Check sheet for the drawn part. Datum: minimum x, y, z corner. Units: mm. Coordinates: 2 decimals unless noted, no trailing zeros. Order: outer loops, then holes, each group sorted by start corner. A loop starts at its lowest first (then second) coordinate and runs counter-clockwise, first axis right, second up. Notation, with made-up numbers: (-32.75, 46) - (24.25, 46) arc R22 cw to (24.25, 57) - close; hole circle Ø3 at (-3, 79.5). An arc over 180 degrees is marked (long way). One line per item, written item: value. Start each with the question number.
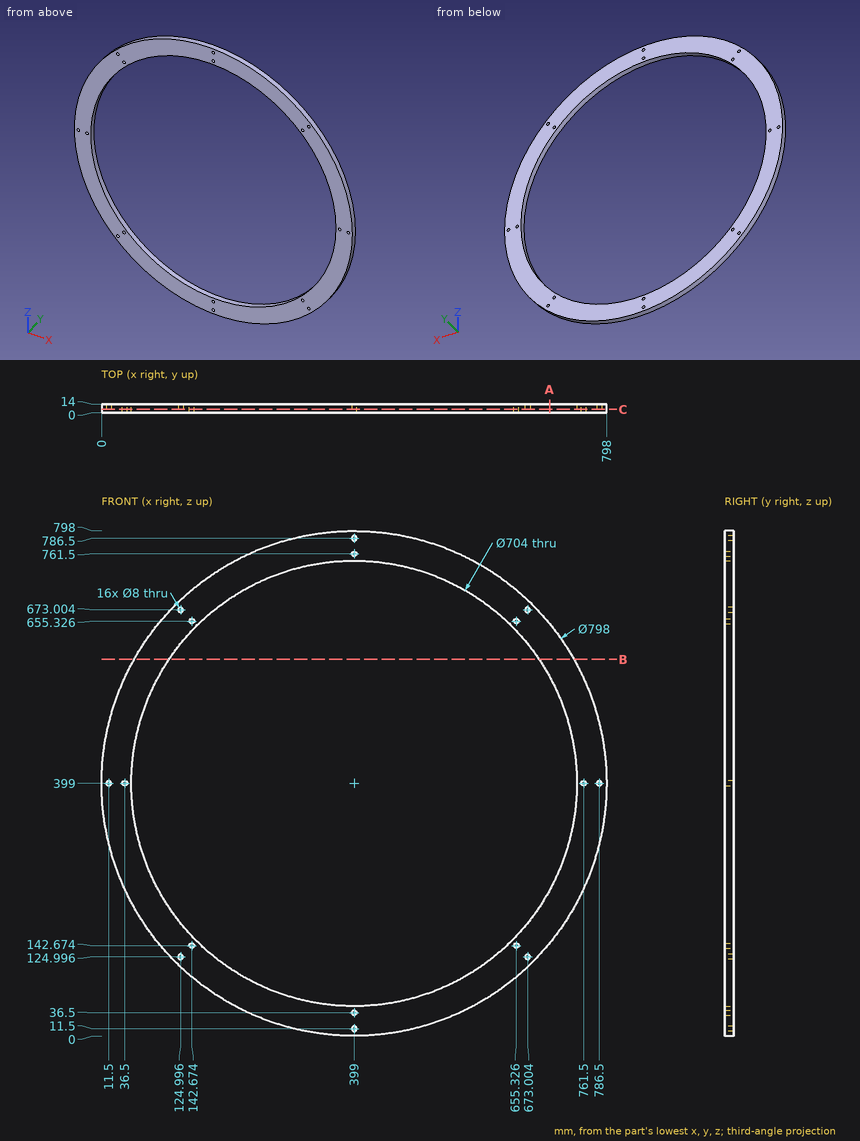
Q1. Material ranges on probe 1 along Z at (x, y) = (399, 5.25); probe 2 along Z at (x, y) = (284.5, 9.25); probe 3 along Z at (x, y) = (541.5, 7), recorded low to high.
Q2. Cross-section at C-C, the plane y = 5.5. Count the separate pieces of the cut face and the enclosed holes in it, and give its area (3 significant figures).
Q3. Cross-section at A-A, the plane x = 708. Enter the section's corners in (y, z), and give its area (3 significant figures).
Q4. Gauge pin test, flat ends, axial feed: P1, Ø6.5, axis at x = 125, z = 673, coming from the +Y side; P2, Ø5, axis at x = 121, y = 11, coming from the -Z side; P3, Ø1, axis at y = 2, z = 351, coming from the +X side; P4, Ø1.5, axis at x = 615, y = 11.5, coming from the -Z side. Record the tip position at first contact, or that the pin passes through.
Q5. Cross-section at B-B, the plane z = 595. Enter the section's corners in (x, y), and give its area (3 significant figures).
Check result:
1. probe 1: z = 0 to 7.5, 15.5 to 32.5, 40.5 to 47, 751 to 757.5, 765.5 to 782.5, 790.5 to 798
1. probe 2: z = 16.78 to 66.14, 731.86 to 781.22
1. probe 3: z = 26.31 to 77.13, 720.87 to 771.69
2. separate pieces: 1
2. enclosed holes: 17
2. area: 110,000 mm2
3. outline: (0, 146.57) - (14, 146.57) - (14, 230.41) - (0, 230.41) - close; (0, 567.59) - (14, 567.59) - (14, 651.43) - (0, 651.43) - close
3. area: 2,350 mm2
4. P1: passes through
4. P2: stops at z = 110.38
4. P3: stops at x = 795.16
4. P4: stops at z = 63.04
5. outline: (51.46, 0) - (106.62, 0) - (106.62, 14) - (51.46, 14) - close; (691.38, 0) - (746.54, 0) - (746.54, 14) - (691.38, 14) - close
5. area: 1,540 mm2
